Source: CAD feature listing. Evaluate the final solid. Frame: model axes, mm. Round coordinates to 2 decimals unless told otherwise and drop trailing zeros. Loops run counter-clockwise (first coordinate to the right, second up) from the corner with the lowest first, then second, coordinate; pieces in that order, holes last.
Item 1: Section query A-A on y = 10. Return loops of the section in (x, z).
Item 2: Ray query, L1, parallel to X at y = 7.75, z = 5; L2, parallel to X at y = 11.75, z = -13; L3, parallel to Y at x = 6.25, z = -25. Return the intervals inside material, ascending.
Item 3: First-contact query: P1, Ø4, axis at x = 11.5, z = -18, coming from the +Y side; P2, Ø8, axis at y = 8, z = -26, coming from the +X side; P3, Ø3, axis at y = 7, z = 24, coming from the -X side; P4, Ø1, axis at x = 6, y = 13.5, coming from the -Z side. Flat tips, straight axial feed; report the tip coordinate or a pass-through.
Item 4: Section query B-B on x = -11.5. Return loops of the section in (y, z), then the cut area to 3 significant figures.
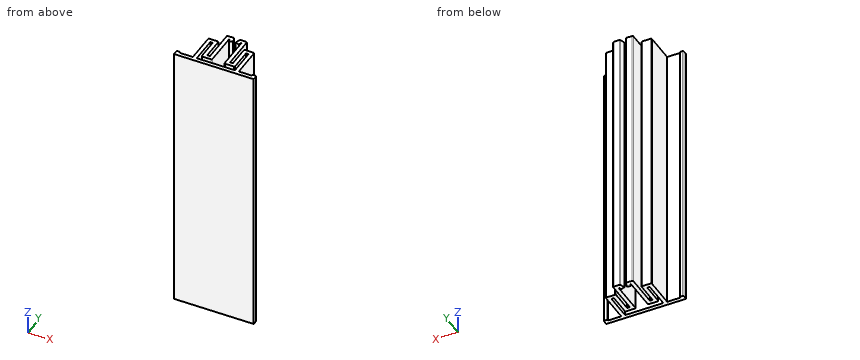
```python
from build123d import *

# Parameters (mm, degrees)
F1_DEPTH = 50
F2_R     = 0.35
F3_R     = 0.35
F4_R     = 0.35
F5_R     = 0.35


with BuildPart() as f1:
    # F0 (on Top) → F1 (new body, symmetric)
    with BuildSketch(Plane.XY):
        Polygon((1.0409717248, 16.8190124818), (0.4387088702, 14.9118471891), (1.7819859847, 14.5164243155), (2.0670138885, 15.4190124818), (2.2409717248, 15.4190124818), (2.2409717248, 3.4190124818), (6.0409717248, 3.4190124818), (6.0409717248, 11.4190124818), (6.9409717248, 11.4190124818), (6.9409717248, 1.8190124818), (-6.9409717248, 1.8190124818), (-6.9409717248, 11.4190124818), (-6.0409717248, 11.4190124818), (-6.0409717248, 3.4190124818), (-2.2409717248, 3.4190124818), (-2.2409717248, 15.4190124818), (-2.0670138885, 15.4190124818), (-1.7819859847, 14.5164243155), (-0.4387088702, 14.9118471891), (-1.0409717248, 16.8190124818), (-3.6409717248, 16.8190124818), (-3.6409717248, 4.8190124818), (-4.6409717248, 4.8190124818), (-4.6409717248, 12.8190124818), (-8.3409717248, 12.8190124818), (-8.3409717248, 1.8190124818), (-13.0909717248, 1.8190124818), (-13.0909717248, 2.3190124818), (-14.4909717248, 2.3190124818), (-14.4909717248, 0.4190124818), (-6.9409717248, 0.4190124818), (6.9409717248, 0.4190124818), (14.4909717248, 0.4190124818), (14.4909717248, 2.3190124818), (13.0909717248, 2.3190124818), (13.0909717248, 1.8190124818), (8.3409717248, 1.8190124818), (8.3409717248, 12.8190124818), (4.6409717248, 12.8190124818), (4.6409717248, 4.8190124818), (3.6409717248, 4.8190124818), (3.6409717248, 16.8190124818), align=None)
    extrude(amount=F1_DEPTH, both=True)

    # F2
    f2_edges = [f1.edges().sort_by_distance(p)[0] for p in [
        (14.490972, 2.319012, 0),
    ]]
    fillet(f2_edges, radius=F2_R)

    # F3
    f3_edges = [f1.edges().sort_by_distance(p)[0] for p in [
        (13.090972, 2.319012, 0),
        (8.340972, 12.819012, 0),
        (4.640972, 12.819012, 0),
        (3.640972, 16.819012, 0),
        (1.040972, 16.819012, 0),
    ]]
    fillet(f3_edges, radius=F3_R)

    # F4
    f4_edges = [f1.edges().sort_by_distance(p)[0] for p in [
        (6.040972, 3.419012, 0),
        (2.240972, 3.419012, 0),
        (-2.240972, 3.419012, 0),
    ]]
    fillet(f4_edges, radius=F4_R)

    # F5
    f5_edges = [f1.edges().sort_by_distance(p)[0] for p in [
        (-6.040972, 3.419012, 0),
        (-8.340972, 12.819012, 0),
        (-14.490972, 2.319012, 0),
        (-3.640972, 16.819012, 0),
        (-1.040972, 16.819012, 0),
        (-4.640972, 12.819012, 0),
        (-13.090972, 2.319012, 0),
    ]]
    fillet(f5_edges, radius=F5_R)


solid = f1.part
```
Data:
1. outline: (-8.34, -50) - (-6.94, -50) - (-6.94, 50) - (-8.34, 50) - close; (-6.04, -50) - (-4.64, -50) - (-4.64, 50) - (-6.04, 50) - close; (-3.64, -50) - (-2.24, -50) - (-2.24, 50) - (-3.64, 50) - close; (2.24, -50) - (3.64, -50) - (3.64, 50) - (2.24, 50) - close; (4.64, -50) - (6.04, -50) - (6.04, 50) - (4.64, 50) - close; (6.94, -50) - (8.34, -50) - (8.34, 50) - (6.94, 50) - close
2. L1: x = -8.34 to -6.94, -6.04 to -4.64, -3.64 to -2.24, 2.24 to 3.64, 4.64 to 6.04, 6.94 to 8.34
2. L2: x = -8.34 to -4.64, -3.64 to -2.24, 2.24 to 3.64, 4.64 to 8.34
2. L3: y = 0.42 to 1.82, 11.42 to 12.82
3. P1: stops at y = 2.32
3. P2: stops at x = 8.34
3. P3: stops at x = -8.34
3. P4: passes through
4. outline: (0.42, -50) - (1.82, -50) - (1.82, 50) - (0.42, 50) - close
4. area: 140 mm2
